from build123d import *

# Parameters (mm, degrees)
ESQUISSE3_W             = 50
ESQUISSE3_H             = 50
BOSS_EXTRU_3_DEPTH      = 3
ESQUISSE4_W             = 8
ESQUISSE4_H             = 35
BOSS_EXTRU_5_DEPTH      = 45
ESQUISSE7_R             = 5
ENL_V_MAT_EXTRU_1_DEPTH = 40
CONG_1_R                = 10
CONG_2_R                = 9.25
CONG_3_R                = 3
D_GAGEMENT_M2_51_D      = 2.7


with BuildPart() as part:
    # Esquisse3 → Boss.-Extru.3 (new body)
    with BuildSketch(Plane(origin=(0, 0, 0), x_dir=(0, 0, -1), z_dir=(1, 0, 0))):
        Rectangle(ESQUISSE3_W, ESQUISSE3_H)
    extrude(amount=BOSS_EXTRU_3_DEPTH)

    # Esquisse4 → Boss.-Extru.5 (add)
    with BuildSketch(Plane(origin=(0, 0, 0), x_dir=(0, 0, -1), z_dir=(1, 0, 0))):
        with Locations((-13.5, 0)):
            Rectangle(ESQUISSE4_W, ESQUISSE4_H)
        with Locations((13.5, 0)):
            Rectangle(ESQUISSE4_W, ESQUISSE4_H)
    extrude(amount=-BOSS_EXTRU_5_DEPTH)

    # Esquisse7 → Enlèv. mat.-Extru.1 (cut)
    with BuildSketch(Plane(origin=(0, 0, -17.5), x_dir=(-1, 0, 0), z_dir=(0, 0, -1))):
        with Locations((30, 0)):
            Circle(ESQUISSE7_R)
    extrude(amount=-ENL_V_MAT_EXTRU_1_DEPTH, mode=Mode.SUBTRACT)

    # Congé1
    # the kernel refuses this fillet: 10 mm, written as the material it adds along each edge
    with BuildSketch(Plane(origin=(0, -17.5, 17.5), x_dir=(0, 0, 1), z_dir=(0, 1, 0))) as cong_1_piece_1:
        with BuildLine():
            CenterArc((10, -9.682458366), CONG_1_R, 104.477512186, 75.522487814)
            Line((0, -9.682458366), (0, 0))
            Line((0, 0), (7.5, 0))
        make_face()
    extrude(amount=35)
    with BuildSketch(Plane(origin=(0, -17.5, -17.5), x_dir=(0, 0, -1), z_dir=(0, 1, 0))) as cong_1_piece_2:
        with BuildLine():
            CenterArc((10, 9.682458366), CONG_1_R, 180, 75.522487814)
            Line((0, 9.682458366), (0, 0))
            Line((0, 0), (7.5, 0))
        make_face()
    extrude(amount=35)
    # the kernel refuses this fillet: 10 mm, written as the material it takes off along each edge
    with BuildSketch(Plane(origin=(-45, 17.5, 42.5), x_dir=(0, -1, 0), z_dir=(0, 0, -1)), Plane(origin=(-45, 17.5, -42.5), x_dir=(1, 0, 0), z_dir=(0, 0, 1))) as cong_1_2_piece_1:
        with BuildLine():
            CenterArc((CONG_1_R, -CONG_1_R), CONG_1_R, 90, 90)
            Line((0, -CONG_1_R), (0, 0))
            Line((0, 0), (CONG_1_R, 0))
        make_face()
    extrude(amount=58, mode=Mode.SUBTRACT)
    with BuildSketch(Plane(origin=(-45, -17.5, -15.5), x_dir=(1, 0, 0), z_dir=(0, 0, 1)), Plane(origin=(-45, -17.5, 15.5), x_dir=(0, 1, 0), z_dir=(0, 0, -1))) as cong_1_2_piece_2:
        with BuildLine():
            CenterArc((CONG_1_R, CONG_1_R), CONG_1_R, 180, 90)
            Line((0, CONG_1_R), (0, 0))
            Line((0, 0), (CONG_1_R, 0))
        make_face()
    extrude(amount=58, mode=Mode.SUBTRACT)

    # Congé2
    cong_2_edges = [part.edges().sort_by_distance(p)[0] for p in [
        (0, 0, 9.5),
        (0, 0, -9.5),
    ]]
    fillet(cong_2_edges, radius=CONG_2_R)

    # Congé3
    cong_3_edges = [part.edges().sort_by_distance(p)[0] for p in [
        (1.5, -25, -25),
        (1.5, -25, 25),
        (1.5, 25, 25),
        (1.5, 25, -25),
    ]]
    fillet(cong_3_edges, radius=CONG_3_R)

    # Dégagement M2.51 (through all)
    with Locations(Plane.ZY):
        with Locations((21, 21.25), (-21, 21.25), (-21, -21.25), (21, -21.25)):
            Hole(D_GAGEMENT_M2_51_D / 2)


solid = part.part
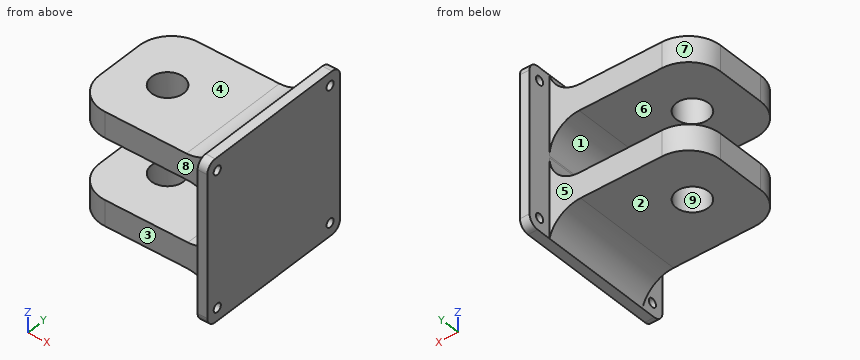
Could you check a few things on this model? Use its own coordinates, in mm. Face numbers are marked on the shaded views. A direction names the side the tool comes from. Coordinates: 2 decimals unless noted, no trailing zeros. Loops run counter-clockwise (first coordinate to the right, second up) from the corner with the lowest first, then second, coordinate; pieces in that order, holes last.
1. I need wall thicknesses on L1, parallel to Y at x = 1.1, z = -21; L2, parallel to Z at x = -3.5, y = 16.5; L3, parallel to Z at x = -9.5, y = 1. Which ranges of each line are inside material? Lowest first, please.
2. Imagine slicing it at B-B (x = -30). Please give me the cut outline in (y, z).
3. We'd pull the mould along Y, two halves only. Please class the marked faces 6, 7, 8 and 9: released by +Y, released by -Y, zero draft, split by the parting line, or undercut.
4. Imagine slicing it at C-C (z = 16). Please give me the cut outline in (x, y), and give its area (3 significant figures).
5. Imagine slicing it at A-A (x = -17.5). Please give me the cut outline in (y, z), and give its area (3 significant figures).
6. Imagine slicing it at D-D (y = 21.25). Please give me the cut outline in (x, z), and give its area (3 significant figures).
7. For P1, Ø10, axis at x = -38, y = 10.5, coming from the -Z side; P2, Ø2, axis at x = -4.5, z = -15.5, coming from the +Y side; P3, Ø3, axis at y = 21.25, z = 21, coming from the -X side, each with a flat end and sliding along its axis, tell me the tip position at first contact or that it passes through.
8. For the marked faces 1, 2, 3, 4 and 5, which set-ups out of +Z, -Z, +X, -X, +Y, -Y let a thin tool reach every point of the face, with its end or its side?
Computed values:
1. L1: y = -25 to -22.6, -19.9 to 19.9, 22.6 to 25
1. L2: z = -19.64 to -7.5, 7.5 to 19.64
1. L3: z = -17.5 to -9.5, 9.5 to 17.5
2. outline: (-17.5, -17.5) - (-5, -17.5) - (-5, -9.5) - (-17.5, -9.5) - close; (-17.5, 9.5) - (-5, 9.5) - (-5, 17.5) - (-17.5, 17.5) - close; (5, -17.5) - (17.5, -17.5) - (17.5, -9.5) - (5, -9.5) - close; (5, 9.5) - (17.5, 9.5) - (17.5, 17.5) - (5, 17.5) - close
3. face 6: zero draft
3. face 7: released by +Y
3. face 8: released by -Y
3. face 9: undercut
4. outline: (-45, -7.5) arc R10 ccw to (-35, -17.5) - (0, -17.5) - (0, -25) - (3, -25) - (3, 25) - (0, 25) - (0, 17.5) - (-35, 17.5) arc R10 ccw to (-45, 7.5) - close; hole circle Ø10 at (-30, 0)
4. area: 1,600 mm2
5. outline: (-17.5, -17.5) - (17.5, -17.5) - (17.5, -9.5) - (-17.5, -9.5) - close; (-17.5, 9.5) - (17.5, 9.5) - (17.5, 17.5) - (-17.5, 17.5) - close
5. area: 560 mm2
6. outline: (0, -25) - (3, -25) - (3, -22.35) - (0, -22.35) - close; (0, -19.65) - (3, -19.65) - (3, 19.65) - (0, 19.65) - close; (0, 22.35) - (3, 22.35) - (3, 25) - (0, 25) - close
6. area: 134 mm2
7. P1: stops at z = -17.5
7. P2: stops at y = 17.5
7. P3: stops at x = 0
8. face 1: -X, +Y, -Y
8. face 2: -Z, -X, +Y, -Y
8. face 3: +Z, -Z, -X, -Y
8. face 4: +Z, -X, +Y, -Y
8. face 5: +Z, -Z, -X, +Y
